from build123d import *

# Parameters (mm, degrees)
BOSS_EXTRUDE1_DEPTH   = 1.5875
SKETCH2_R             = 6.35
SKETCH2_R_2           = 5.715
SKETCH2_W             = 11.94
SKETCH2_H             = 20.64
SKETCH2_W_2           = 14.605
SKETCH2_H_2           = 14.605
SKETCH2_W_3           = 45.462
SKETCH2_H_3           = 102.32
CUT_EXTRUDE1_DEPTH    = 2.5875
F_6_CLEARANCE_HOLE2_D = 4.3053
CUT_EXTRUDE2_START    = -1.5875
SKETCH7_W             = 13.332833865
SKETCH7_H             = 14.312726798
SKETCH7_W_2           = 13.529020254
SKETCH7_H_2           = 14.424558237
CUT_EXTRUDE2_DEPTH    = 1.5875


with BuildPart() as part:
    # Sketch1 → Boss-Extrude1 (new body)
    with BuildSketch(Plane.XY):
        with BuildLine():
            Line((58.206752076, 169.534029068), (58.206752076, 175.566529068))
            Line((58.206752076, 175.566529068), (-81.493247924, 175.566529068))
            Line((-81.493247924, 175.566529068), (-81.493247924, 169.534029068))
            ThreePointArc((-81.493247924, 169.534029068), (-82.981145475, 165.941926619), (-86.573247924, 164.454029068))
            Line((-86.573247924, 164.454029068), (-98.161997924, 164.454029068))
            Line((-98.161997924, 164.454029068), (-98.161997924, 61.266529068))
            Line((-98.161997924, 61.266529068), (74.875502076, 61.266529068))
            Line((74.875502076, 61.266529068), (74.875502076, 164.454029068))
            Line((74.875502076, 164.454029068), (63.286752076, 164.454029068))
            ThreePointArc((63.286752076, 164.454029068), (59.694649628, 165.941926619), (58.206752076, 169.534029068))
        make_face()
    extrude(amount=BOSS_EXTRUDE1_DEPTH)

    # Sketch2 → Cut-Extrude1 (cut, through all)
    with BuildSketch(Plane.XY.offset(1.5875)):
        with Locations((-84.668247924, 152.389029068)):
            Circle(SKETCH2_R)
        with Locations((-84.668247924, 107.304029068)):
            Circle(SKETCH2_R)
        with Locations((63.540752076, 132.386529068)):
            Circle(SKETCH2_R)
        with Locations((62.651752076, 107.304029068)):
            Circle(SKETCH2_R)
        with Locations((-18.374247924, 77.776529068)):
            Circle(SKETCH2_R_2)
        with Locations((-18.374247924, 98.096529068)):
            Circle(SKETCH2_R_2)
        with Locations((-18.374247924, 118.416529068)):
            Circle(SKETCH2_R_2)
        with Locations((-18.374247924, 138.736529068)):
            Circle(SKETCH2_R_2)
        with Locations((-18.374247924, 159.056529068)):
            Circle(SKETCH2_R_2)
        with Locations((63.286752076, 152.706529068)):
            Circle(SKETCH2_R_2)
        with Locations((62.016752076, 77.649529068)):
            Rectangle(SKETCH2_W, SKETCH2_H)
        with Locations((39.791752076, 80.316529068)):
            Rectangle(SKETCH2_W_2, SKETCH2_H_2)
        with Locations((39.791752076, 99.112529068)):
            Rectangle(SKETCH2_W_2, SKETCH2_H_2)
        with Locations((39.791752076, 117.908529068)):
            Rectangle(SKETCH2_W_2, SKETCH2_H_2)
        with Locations((20.995752076, 80.316529068)):
            Rectangle(SKETCH2_W_2, SKETCH2_H_2)
        Polygon((32.489252076, 141.609529068), (32.489252076, 129.402029068), (47.094252076, 129.402029068), (47.094252076, 141.609529068), (54.396752076, 141.609529068), (54.396752076, 170.249529068), (-11.643247924, 170.249529068), (-11.643247924, 141.609529068), (-5.102747924, 141.609529068), (-5.102747924, 129.402029068), (9.502252076, 129.402029068), (9.502252076, 141.609529068), (13.693252076, 141.609529068), (13.693252076, 129.402029068), (28.298252076, 129.402029068), (28.298252076, 141.609529068), align=None)
        with Locations((20.995752076, 99.112529068)):
            Rectangle(SKETCH2_W_2, SKETCH2_H_2)
        with Locations((20.995752076, 117.908529068)):
            Rectangle(SKETCH2_W_2, SKETCH2_H_2)
        with Locations((2.199752076, 117.908529068)):
            Rectangle(SKETCH2_W_2, SKETCH2_H_2)
        with Locations((2.199752076, 99.112529068)):
            Rectangle(SKETCH2_W_2, SKETCH2_H_2)
        with Locations((2.199752076, 80.316529068)):
            Rectangle(SKETCH2_W_2, SKETCH2_H_2)
        with Locations((-85.303247924, 132.386529068)):
            Rectangle(SKETCH2_W_2, SKETCH2_H_2)
        with Locations((-51.442247924, 118.289529068)):
            Rectangle(SKETCH2_W_3, SKETCH2_H_3)
        with Locations((-85.303247924, 77.649529068)):
            Rectangle(SKETCH2_W, SKETCH2_H)
    extrude(amount=-CUT_EXTRUDE1_DEPTH, mode=Mode.SUBTRACT)

    # #6 Clearance Hole2 (through all)
    with Locations(Plane(origin=(-11.643247924, -6.662700632, -3.175), x_dir=(-1, 0, 0), z_dir=(0, 0, -1))):
        with Locations((-81.28, 124.6982297), (6.731, 175.8792297), (81.28, 124.6982297), (6.731, 74.2792297)):
            Hole(F_6_CLEARANCE_HOLE2_D / 2)

    # Sketch7 → Cut-Extrude2 (cut)
    with BuildSketch(Plane.XY.offset(1.5875).offset(CUT_EXTRUDE2_START)):
        with Locations((62.004967044, 77.673806769)):
            Rectangle(SKETCH7_W, SKETCH7_H)
        with Locations((-85.255785181, 77.616484213)):
            Rectangle(SKETCH7_W_2, SKETCH7_H_2)
    extrude(amount=CUT_EXTRUDE2_DEPTH, mode=Mode.SUBTRACT)


solid = part.part
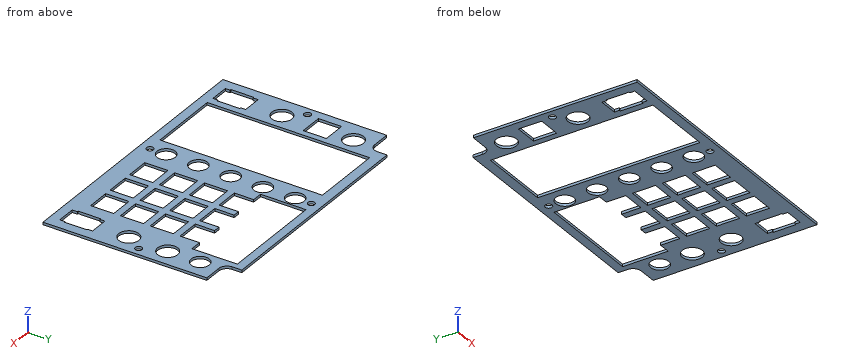
Model file for the job. Use its own axes, mm. Coordinates: 2 decimals unless noted, no trailing zeros. Write each loop counter-clockwise with the first axis right and the second up, starting at its lowest first coordinate (ties: lowest second). Pieces come first, ordered by that corner, then holes. Notation, with made-up numbers: (40.5, -7.75) - (93.5, -7.75) arc R18 ccw to (93.5, 16.25) - close; hole circle Ø2 at (-34, 7.5). An arc over 180 degrees is marked (long way). Write each question's results on one line, items separated by ' | '. Start each with the question number.
1) Flat gauge pins, fed straight in: P1, Ø0.8, axis at x = 71, z = 0.5, coming from the +Y side; P2, Ø5, axis at x = -92.92, y = 118.04, coming from the +Z side. Where does each tip first touch, or does it go through?
2) Probe line 1 along Y through (x, z) = (44.5, 1); line 2 along X through (y, z) = (153, 0.1); line 3 along X through (y, z) = (91.5, 0.55). List the from-to ranges inside material, lowest first. Write a range as from..to.
3) Cut at D-D (z = 0.5). Count the separate pieces of the cut face and the enclosed holes in it, then the cut area to 3 significant figures.
4) Cut at B-B (y = 156.5). Write the cut outline in (x, z), then the cut area to 3 significant figures.
5) Cut at A-A (x = -65). Write the cut outline in (y, z).
6) Cut at C-C (x = 61). Write the cut outline in (y, z).
Returned:
1) P1: y = 164.45 | P2: z = 1.59
2) line 1: 61.27..73.01, 87.62..91.81, 106.42..110.61, 125.21..129.4, 170.25..175.57 | line 2: -98.16..-90.99, -78.35..-74.17, -28.71..-11.64, 54.4..57.58, 68.99..74.88 | line 3: -98.16..-74.17, -28.71..74.88
3) separate pieces: 1 | enclosed holes: 28 | area: 8,490 mm^2
4) outline: (-98.16, 0) - (-89.51, 0) - (-89.51, 1.59) - (-98.16, 1.59) - close; (-79.83, 0) - (-74.17, 0) - (-74.17, 1.59) - (-79.83, 1.59) - close; (-28.71, 0) - (-23.49, 0) - (-23.49, 1.59) - (-28.71, 1.59) - close; (-13.26, 0) - (-11.64, 0) - (-11.64, 1.59) - (-13.26, 1.59) - close; (54.4, 0) - (59.01, 0) - (59.01, 1.59) - (54.4, 1.59) - close; (67.56, 0) - (74.88, 0) - (74.88, 1.59) - (67.56, 1.59) - close | area: 52.5 mm^2
5) outline: (61.27, 0) - (67.13, 0) - (67.13, 1.59) - (61.27, 1.59) - close; (169.45, 0) - (175.57, 0) - (175.57, 1.59) - (169.45, 1.59) - close
6) outline: (61.27, 0) - (67.33, 0) - (67.33, 1.59) - (61.27, 1.59) - close; (87.97, 0) - (101.17, 0) - (101.17, 1.59) - (87.97, 1.59) - close; (113.44, 0) - (126.57, 0) - (126.57, 1.59) - (113.44, 1.59) - close; (138.21, 0) - (147.47, 0) - (147.47, 1.59) - (138.21, 1.59) - close; (157.94, 0) - (165, 0) - (165, 1.59) - (157.94, 1.59) - close
